The model under review builds one solid part; all positions refer to its coordinate system, in mm. A direction names the side the tool comes from. Give positions to 0.01 mm unless a question says otherwise; leave off trailing zeros. Order: outer loops, then holes, each group sorted by start corner. A loop starts at its lowest first (then second) coordinate and runs counter-clockwise, first axis right, second up. Notation, with made-up numbers: (71.5, 83) - (130.5, 83) arc R34 cw to (130.5, 117) - close; hole circle Ø10 at (-33, 43). An arc over 180 degrees is marked (long way). Use a Markdown table: item, result. Add a question column.
```python
from build123d import *

# Parameters (mm, degrees)
F0_R     = 1.175
F1_DEPTH = 0.79375


with BuildPart() as f1:
    # F0 (on Top) → F1 (new body)
    with BuildSketch(Plane.XY):
        with BuildLine():
            Line((-95.623562, 91.834139), (-95.623562, 90.626995))
            Line((-95.623562, 90.626995), (-85.873562, 29.398428))
            Line((-85.873562, 29.398428), (-84.167312, 29.398428))
            ThreePointArc((-84.167312, 29.398428), (-83.606046, 29.165944), (-83.373562, 28.604678))
            Line((-83.373562, 28.604678), (-83.373562, 7.192178))
            ThreePointArc((-83.373562, 7.192178), (-83.141078, 6.630911), (-82.579812, 6.398428))
            Line((-82.579812, 6.398428), (-81.873562, 6.398428))
            Line((-81.873562, 6.398428), (-74.314535, -27.775555))
            Line((-74.314535, -27.775555), (-71.108285, -27.775555))
            ThreePointArc((-71.108285, -27.775555), (-70.547019, -28.008039), (-70.314535, -28.569305))
            Line((-70.314535, -28.569305), (-70.314535, -39.775555))
            Line((-70.314535, -39.775555), (-51.43259, -39.775555))
            Line((-51.43259, -39.775555), (-51.43259, -28.569305))
            ThreePointArc((-51.43259, -28.569305), (-51.200106, -28.008039), (-50.63884, -27.775555))
            Line((-50.63884, -27.775555), (-47.43259, -27.775555))
            Line((-47.43259, -27.775555), (-40.011215, 5.776105))
            ThreePointArc((-40.011215, 5.776105), (-39.733173, 6.223592), (-39.236198, 6.398428))
            Line((-39.236198, 6.398428), (-39.167312, 6.398428))
            ThreePointArc((-39.167312, 6.398428), (-38.606046, 6.630911), (-38.373562, 7.192178))
            Line((-38.373562, 7.192178), (-38.373562, 28.604678))
            ThreePointArc((-38.373562, 28.604678), (-38.141078, 29.165944), (-37.579812, 29.398428))
            Line((-37.579812, 29.398428), (-36.550917, 29.398428))
            ThreePointArc((-36.550917, 29.398428), (-36.035669, 29.58839), (-35.767043, 30.067354))
            Line((-35.767043, 30.067354), (-26.123562, 90.626995))
            Line((-26.123562, 90.626995), (-26.123562, 91.834139))
            ThreePointArc((-26.123562, 91.834139), (-29.052495, 98.905207), (-36.123562, 101.834139))
            Line((-36.123562, 101.834139), (-36.267312, 101.834139))
            ThreePointArc((-36.267312, 101.834139), (-36.828578, 102.066623), (-37.061062, 102.627889))
            Line((-37.061062, 102.627889), (-37.061062, 103.041283))
            ThreePointArc((-37.061062, 103.041283), (-39.989995, 110.112351), (-47.061062, 113.041283))
            Line((-47.061062, 113.041283), (-47.379812, 113.041283))
            ThreePointArc((-47.379812, 113.041283), (-47.941078, 113.273767), (-48.173562, 113.835033))
            Line((-48.173562, 113.835033), (-48.173562, 116.248428))
            ThreePointArc((-48.173562, 116.248428), (-50.516708, 121.905282), (-56.173562, 124.248428))
            Line((-56.173562, 124.248428), (-65.573562, 124.248428))
            ThreePointArc((-65.573562, 124.248428), (-71.230417, 121.905282), (-73.573562, 116.248428))
            Line((-73.573562, 116.248428), (-73.573562, 113.835033))
            ThreePointArc((-73.573562, 113.835033), (-73.806046, 113.273767), (-74.367312, 113.041283))
            Line((-74.367312, 113.041283), (-74.686062, 113.041283))
            ThreePointArc((-74.686062, 113.041283), (-81.75713, 110.112351), (-84.686062, 103.041283))
            Line((-84.686062, 103.041283), (-84.686062, 102.627889))
            ThreePointArc((-84.686062, 102.627889), (-84.918546, 102.066623), (-85.479812, 101.834139))
            Line((-85.479812, 101.834139), (-85.623562, 101.834139))
            ThreePointArc((-85.623562, 101.834139), (-92.69463, 98.905207), (-95.623562, 91.834139))
        make_face()
        with Locations((-78.657184, 8.448236)):
            Circle(F0_R, mode=Mode.SUBTRACT)
        with Locations((-60.873562, -31.726764)):
            Circle(F0_R, mode=Mode.SUBTRACT)
        with BuildLine():
            Line((-67.829812, -18.051764), (-53.917312, -18.051764))
            ThreePointArc((-53.917312, -18.051764), (-53.356046, -18.284248), (-53.123562, -18.845514))
            Line((-53.123562, -18.845514), (-53.123562, -20.258014))
            ThreePointArc((-53.123562, -20.258014), (-53.356046, -20.81928), (-53.917312, -21.051764))
            Line((-53.917312, -21.051764), (-67.829812, -21.051764))
            ThreePointArc((-67.829812, -21.051764), (-68.391078, -20.81928), (-68.623562, -20.258014))
            Line((-68.623562, -20.258014), (-68.623562, -18.845514))
            ThreePointArc((-68.623562, -18.845514), (-68.391078, -18.284248), (-67.829812, -18.051764))
        make_face(mode=Mode.SUBTRACT)
        with BuildLine():
            Line((-69.579812, -9.051764), (-52.167312, -9.051764))
            ThreePointArc((-52.167312, -9.051764), (-51.606046, -9.284248), (-51.373562, -9.845514))
            Line((-51.373562, -9.845514), (-51.373562, -14.258014))
            ThreePointArc((-51.373562, -14.258014), (-51.606046, -14.81928), (-52.167312, -15.051764))
            Line((-52.167312, -15.051764), (-69.579812, -15.051764))
            ThreePointArc((-69.579812, -15.051764), (-70.141078, -14.81928), (-70.373562, -14.258014))
            Line((-70.373562, -14.258014), (-70.373562, -9.845514))
            ThreePointArc((-70.373562, -9.845514), (-70.141078, -9.284248), (-69.579812, -9.051764))
        make_face(mode=Mode.SUBTRACT)
        with BuildLine():
            Line((-73.873562, 30.192178), (-73.873562, 86.548428))
            Line((-73.873562, 86.548428), (-47.873562, 86.548428))
            Line((-47.873562, 86.548428), (-47.873562, 30.192178))
            ThreePointArc((-47.873562, 30.192178), (-47.641078, 29.630911), (-47.079812, 29.398428))
            Line((-47.079812, 29.398428), (-46.667312, 29.398428))
            ThreePointArc((-46.667312, 29.398428), (-46.106046, 29.165944), (-45.873562, 28.604678))
            Line((-45.873562, 28.604678), (-45.873562, 13.523428))
            Line((-45.873562, 13.523428), (-49.623409, -3.429442))
            ThreePointArc((-49.623409, -3.429442), (-49.901452, -3.876928), (-50.398426, -4.051764))
            Line((-50.398426, -4.051764), (-71.348698, -4.051764))
            ThreePointArc((-71.348698, -4.051764), (-71.845673, -3.876928), (-72.123715, -3.429442))
            Line((-72.123715, -3.429442), (-75.873562, 13.523428))
            Line((-75.873562, 13.523428), (-75.873562, 28.604678))
            ThreePointArc((-75.873562, 28.604678), (-75.641078, 29.165944), (-75.079812, 29.398428))
            Line((-75.079812, 29.398428), (-74.667312, 29.398428))
            ThreePointArc((-74.667312, 29.398428), (-74.106046, 29.630911), (-73.873562, 30.192178))
        make_face(mode=Mode.SUBTRACT)
        with Locations((-43.08994, 8.448236)):
            Circle(F0_R, mode=Mode.SUBTRACT)
    extrude(amount=F1_DEPTH)


solid = f1.part
```
Q1. Wall thickness on probe 1 along Y at (x, z) = (-59, 0.75); probe 2 along Y at (x, z) = (-52, 0.4); probe 3 along X at (y, z) = (8, 0.2): over which ranges is each line inside the solid? List them lowest first.
Q2. Machinability: for faces 4 (the flat face through (-47.72, 5.17, 0.39)), 5 (the cylindrical face through (-92.6, 99, 0.4)), which of the approach directions +Z, -Z, +X, -X, +Y, -Y give a long, thin tool a straight path to every point of the face, cutting with its end or side? Answer none if there is none.
Q3. We need section A-A (y = 20.5). Write out the cut boundary in (x, z).
Q4. We need section B-B (y = 85). Write out the cut boundary in (x, z), plus the area to 3 significant figures.
Q5. We need section C-C (z = 0.2). Count the separate pieces of the cut face and the enclosed holes in it, plus the area to 3 significant figures.
Q6. Draft analysis for pull direction Y (two halves, no side actions). For faces 1 (the flat face through (-90.817, 60.441, 0.391)), 2 (the cylindrical face through (-39.91, 110.03, 0.39)), 3 (the flat face through (-73.972, 4.928, 0.391)), state which applies: pulls with the +Y half, pulls with the -Y half, needs draft (parallel to the pull), parting line crosses it, or undercut.
Here are the results:
| question | item | result |
|---|---|---|
| 1 | probe 1 | -39.78 to -21.05, -18.05 to -15.05, -9.05 to -4.05, 86.55 to 124.25 |
| 1 | probe 2 | -39.78 to -15.03, -9.07 to -4.05, 86.55 to 123.07 |
| 1 | probe 3 | -83.37 to -79.74, -77.57 to -74.65, -47.1 to -44.18, -42 to -38.37 |
| 2 | face 4 | +Z, -Z |
| 2 | face 5 | +Z, -Z, -X, +Y |
| 3 | outline | (-83.37, 0) - (-75.87, 0) - (-75.87, 0.79) - (-83.37, 0.79) - close; (-45.87, 0) - (-38.37, 0) - (-38.37, 0.79) - (-45.87, 0.79) - close |
| 4 | outline | (-94.73, 0) - (-73.87, 0) - (-73.87, 0.79) - (-94.73, 0.79) - close; (-47.87, 0) - (-27.02, 0) - (-27.02, 0.79) - (-47.87, 0.79) - close |
| 4 | area | 33.1 mm2 |
| 5 | separate pieces | 1 |
| 5 | enclosed holes | 6 |
| 5 | area | 4,990 mm2 |
| 6 | face 1 | pulls with the -Y half |
| 6 | face 2 | pulls with the +Y half |
| 6 | face 3 | undercut |
